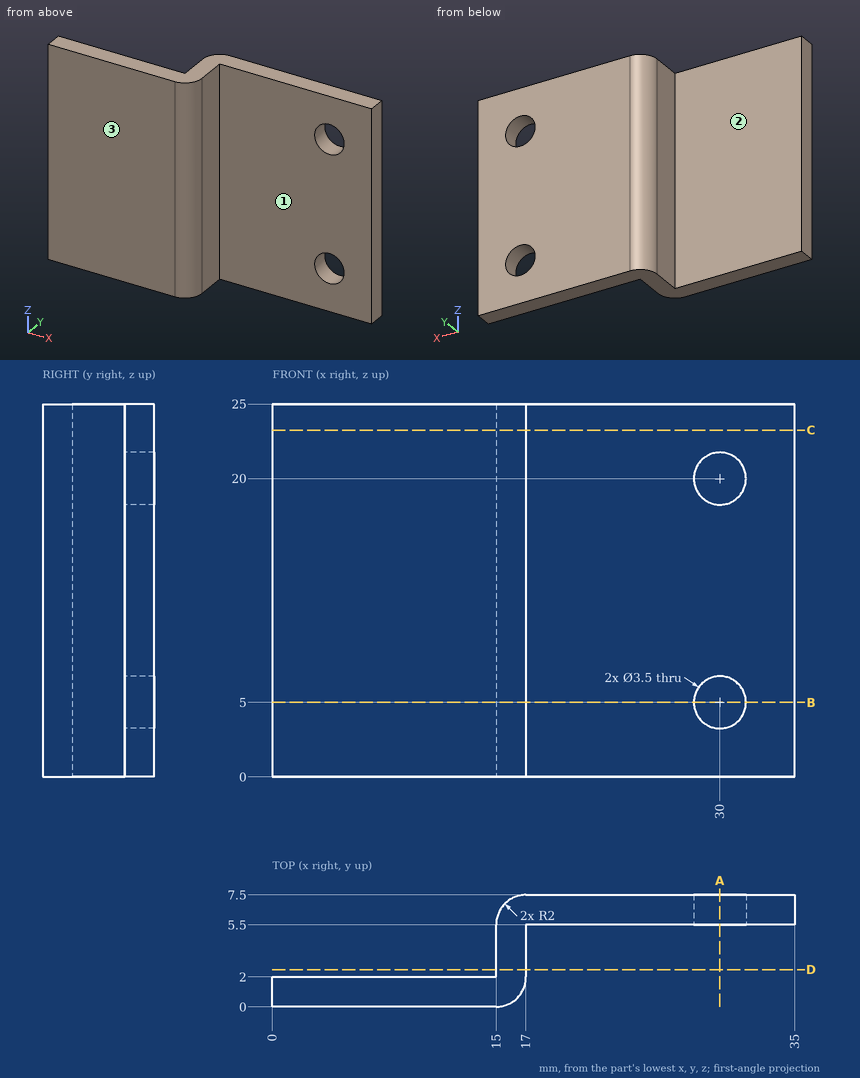
Study the drawing (mm; zero at the part's minimum x, y, z) and answer. A direction names the side the tool comes from. Coordinates: 2 decimals unless noted, no trailing zeros. Loops run counter-clockwise (first coordinate to the right, second up) from the corner with the lowest first, then second, coordinate; pieces in that order, holes last. Notation, with made-up numbers: (-33.75, 10.5) -> (-26.75, 10.5) arc R13 cw to (-26.75, 33.5) -> close; hole circle Ø10 at (30.5, 26). An arc over 180 degrees is marked (long way). Write item = value, one per line. Start each with the question number.
1) The part is cut by section B-B, the plane z = 5. Determine the outline of the cut face in (x, y), plus the area to 3 significant figures.
2) The part is cut by section D-D, the plane y = 2.5. Determine the outline of the cut face in (x, z), plus the area to 3 significant figures.
3) The part is cut by section C-C, the plane z = 23.25. Determine the outline of the cut face in (x, y).
4) The part is cut by section A-A, the plane x = 30. Determine the outline of the cut face in (y, z), plus the area to 3 significant figures.
5) Given P1, Ø5, axis at x = 24.5, z = 7.5, coming from the -Y side; P2, Ø4, axis at y = 3.5, z = 14.5, coming from the -X side; P3, Ø1, axis at y = 3, z = 17, coming from the +X side; P4, Ø14.5, axis at x = 23, z = 14.5, coming from the -Y side, each flat-ended and moving along its own axis, determine where each tip first touches the part or whether it passes through.
6) For the marked faces 1, 2 and 3, determine the directions among +Z, -Z, +X, -X, +Y, -Y from which every point of the face is accessible in a straight line to the end or side of a thin tool.
7) Find the intervals of material crossed by L1, parallel to Z at x = 30, y = 6.6; L2, parallel to X at y = 2.25, z = 14; L3, parallel to Y at x = 4, z = 3.75, in increasing order. Write a range as from..to.
Result:
q1.outline = (0, 0) -> (15, 0) arc R2 ccw to (17, 2) -> (17, 5.5) -> (28.25, 5.5) -> (28.25, 7.5) -> (17, 7.5) arc R2 ccw to (15, 5.5) -> (15, 2) -> (0, 2) -> close; (31.75, 5.5) -> (35, 5.5) -> (35, 7.5) -> (31.75, 7.5) -> close
q1.area = 72.3 mm²
q2.outline = (15, 0) -> (17, 0) -> (17, 25) -> (15, 25) -> close
q2.area = 50.0 mm²
q3.outline = (0, 0) -> (15, 0) arc R2 ccw to (17, 2) -> (17, 5.5) -> (35, 5.5) -> (35, 7.5) -> (17, 7.5) arc R2 ccw to (15, 5.5) -> (15, 2) -> (0, 2) -> close
q4.outline = (5.5, 0) -> (7.5, 0) -> (7.5, 3.25) -> (5.5, 3.25) -> close; (5.5, 6.75) -> (7.5, 6.75) -> (7.5, 18.25) -> (5.5, 18.25) -> close; (5.5, 21.75) -> (7.5, 21.75) -> (7.5, 25) -> (5.5, 25) -> close
q4.area = 36.0 mm²
q5.P1 = 5.5
q5.P2 = 0
q5.P3 = 17
q5.P4 = 0.15
q6.face_1 = +Z, -Z, +X, -Y
q6.face_2 = +Z, -Z, -X, +Y
q6.face_3 = +Z, -Z, +X, -X, -Y
q7.L1 = 0..3.25, 6.75..18.25, 21.75..25
q7.L2 = 15..17
q7.L3 = 0..2
